Source: CAD feature listing. Evaluate the final solid. Frame: model axes, mm. Coordinates: 2 decimals unless noted, no trailing zeros. Write each loop counter-clockwise with the first axis right and the second up, starting at its lowest first coordinate (ties: lowest second). Pieces come first, ordered by that corner, then holes. Notation, with made-up numbers: M 65.25,-30 L 101.25,-30 A8 cw 101.25,-21 Z; hole C -8,43 d6. An arc over 180 degrees is marked long. Write item = value, one per line. Start each with the question number.
1. Section query A-A (y = -6). Output: boundary loops of the cut face in (x, z), then the cut area to 3 significant figures.
2. Line query: line 1 along Z through (x, y) = (-4.25, -6); line 2 along X through (y, z) = (-2.4, -22); line 3 along Y through (x, z) = (-1.5, -15.5). Output: solid intervals per line, ascending.
3. Section query C-C (z = -22). Output: boundary loops of the cut face in (x, y).
4. Pull-direction query (X, two-part tool) for faces 1 (the face through (-2.58, -9.69, -22.33)), 2 (the face through (-7.9, -3, -14)), 3 (the face through (-3.9, -4.8, -7.6)); classes: pulls with the +X half, pulls with the -X half, needs draft (parallel to the pull), parting line crosses it, or undercut.
5. Section query D-D (z = -14). Output: boundary loops of the cut face in (x, y), then the cut area to 3 significant figures.
6. Section query B-B (x = -2.25). Output: boundary loops of the cut face in (y, z).
Autodesk Inventor part; units mm, degrees
ref_plane "YZ Plane" through (0, 0, 0) normal (1, 0, 0) x (0, 1, 0)
ref_plane "XZ Plane" through (0, 0, 0) normal (0, 1, 0) x (-1, 0, 0)
ref_plane "XY Plane" through (0, 0, 0) normal (0, 0, 1) x (1, 0, 0)
sketch "Sketch1" plane through (0, 0, 0) normal (0, 1, 0) x (-1, 0, 0)
  line L0 (0, 0) -> (7.9, 0)
  line L1 (7.9, 0) -> (7.9, -28)
  line L2 (7.9, -28) -> (0, -28)
  line L3 (0, -28) -> (0, 0)
  dimension "d0" = 7.9
  dimension "d1" = 28
extrude "Extrusion1" add sketch "Sketch1" against normal blind 12
sketch "Sketch2" plane through (0, 0, 0) normal (0, 1, 0) x (1, 0, 0)
  line L0 (0, 0) -> (-7.9, 0)
  line L1 (-7.9, 28) -> (0, 28)
  point P0 (-4.043, 6)
  point P1 (-4.043, 22)
  dimension "d4" = 6
  dimension "d5" = 6
hole "Hole1" at (-4.043, 0, -6) at (-4.043, 0, -22) direction (0, -1, 0) diameter 3 end through all
sketch "Sketch3" plane through (-7.9, 0, -28) normal (-1, 0, 0) x (0, 0, 1)
  line L0 (28, 0) -> (28, -12)
  point P0 (22, -6)
  point P1 (14, -6)
  point P2 (6, -6)
  point P3 (28, -6)
  dimension "d13" = 6
  dimension "d14" = 8
  dimension "d15" = 8
hole "Hole2" at (-7.9, -6, -6) at (-7.9, -6, -14) at (-7.9, -6, -22) direction (1, 0, 0) diameter 4 end through all
properties part number "09-0004" material "Aluminum 6061"
Results are:
q1.outline = M -7.9,-28 L 0,-28 L 0,-24 L -7.9,-24 Z; M -7.9,-20 L 0,-20 L 0,-16 L -7.9,-16 Z; M -7.9,-12 L 0,-12 L 0,-8 L -7.9,-8 Z; M -7.9,-4 L 0,-4 L 0,0 L -7.9,0 Z
q1.area = 126 mm^2
q2.line_1 = -28 to -24, -20 to -16, -12 to -8, -4 to 0
q2.line_2 = -7.9 to -5.54, -2.54 to 0
q2.line_3 = -12 to -7.32, -4.68 to 0
q3.outline = M -7.9,-12 L -5.54,-12 L -5.54,-8 L -7.9,-8 Z; M -7.9,-4 L -5.54,-4 L -5.54,0 L -7.9,0 Z; M -2.54,-12 L 0,-12 L 0,-8 L -2.54,-8 Z; M -2.54,-4 L 0,-4 L 0,0 L -2.54,0 Z
q4.face_1 = undercut
q4.face_2 = pulls with the -X half
q4.face_3 = needs draft
q5.outline = M -7.9,-12 L 0,-12 L 0,-8 L -7.9,-8 Z; M -7.9,-4 L 0,-4 L 0,0 L -7.9,0 Z
q5.area = 63.2 mm^2
q6.outline = M -12,-28 L 0,-28 L 0,0 L -12,0 Z; hole C -6,-22 d4; hole C -6,-14 d4; hole C -6,-6 d4
